Can you work these out from the model? Positions are in its coordinate system, mm. Face numbers are marked on the shaded views. A direction names the side the tool comes from. Coordinates: 2 decimals unless noted, no trailing zeros. Order: outer loops, then holes, each group sorted by start corner. A loop starts at its lowest first (then second) coordinate and runs counter-clockwise, first axis right, second up.
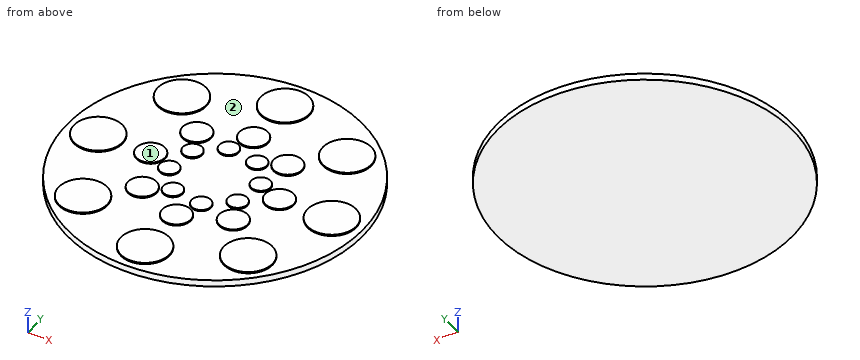
```python
from build123d import *

# Parameters (mm, degrees)
F0_R     = 225
F1_DEPTH = 10
F2_R     = 36.9864384412
F2_R_2   = 21.7454824125
F2_R_3   = 14.7171600395
F3_DEPTH = 2
F5_COUNT = 8


with BuildPart() as f1:
    # F0 (on Top) → F1 (new body)
    with BuildSketch(Plane.XY):
        Circle(F0_R)
    extrude(amount=F1_DEPTH)

    # F2 (on face) → F3 (join)
    with BuildSketch(Plane.XY.offset(10)):
        with Locations((0, 178.0137121677)):
            Circle(F2_R)
        with Locations((0, 98.1170013547)):
            Circle(F2_R_2)
        with Locations((-15.2443298139, 60.619816184)):
            Circle(F2_R_3)
    extrude(amount=F3_DEPTH)

    # F5: F1 ×8 about axis
    f5_axis = Axis((0, 0, 41.8870747089), (0, 0, 1))


with BuildPart() as f1_1:
    add(f1.part)
    for i in range(1, F5_COUNT):
        add(f1.part.rotate(f5_axis, i * 360 / F5_COUNT))


solid = f1_1.part
```
1. Imagine slicing it at A-A on x = -10. Please give me the cut outline in (y, z), then the cut area to 3 significant figures.
Completed:
outline: (-224.78, 0) - (224.78, 0) - (224.78, 10) - (213.62, 10) - (213.62, 12) - (142.4, 12) - (142.4, 10) - (117.43, 10) - (117.43, 12) - (78.81, 12) - (78.81, 10) - (74.37, 10) - (74.37, 12) - (46.87, 12) - (46.87, 10) - (-78.81, 10) - (-78.81, 12) - (-117.43, 12) - (-117.43, 10) - (-142.4, 10) - (-142.4, 12) - (-213.62, 12) - (-213.62, 10) - (-224.78, 10) - close
area: 4,990 mm2
2. On a 3-axis mill with a long thin cutter (end or side, diameter ignored), from which of +Z, -Z, +X, -X, +Y, -Y can I reach the whole of each face in a straight line? I mean the marked faces 1 and 2. Say none if no direction works.
Completed:
face 1: +Z, +X, -X, +Y, -Y
face 2: +Z
3. Please list where these lines run through material, in increasing order: probe 1 along X at (y, z) = (-114, 10.25); probe 2 along Z at (x, y) = (-156, 97); probe 3 along X at (y, z) = (-5.5, 7.25).
Completed:
probe 1: x = -160.9 to -90.85, -14.85 to 14.85, 90.85 to 160.9
probe 2: z = 0 to 10
probe 3: x = -224.93 to 224.93
4. I'm going to push flat-ended pins straight in: pin 1 (1 mm diameter, centred on y = -145, z = 8, fed in from -X); pin 2 (4 mm diameter, centred on x = 94, z = 3.5, fed in from -Y); pin 3 (4 mm diameter, centred on x = -165, y = 77.5, fed in from +Z). Where does each tip first touch, or does it pass through?
Completed:
pin 1: stops at x = -172.47
pin 2: stops at y = -205.33
pin 3: stops at z = 10
